Work out the finished part from the listing and answer in its coordinate system (mm). A direction names the side the tool comes from. Round coordinates to 2 decimals unless told otherwise and drop trailing zeros. Order: outer loops, then holes, each group sorted by start corner. A loop starts at its lowest first (then second) coordinate and runs counter-clockwise, first axis right, second up. Notation, with made-up numbers: M 83.5,2.5 L 129.5,2.5 A20 ccw 129.5,30.5 Z; hole C 65,38 d7. An arc over 180 degrees is marked long. Return JSON: item names as keys, results as strings.
from build123d import *

# Parameters (mm, degrees)
SKETCH_3_R          = 1.6
EXTRUDE_2_DEPTH     = 3
SKETCH_4_W          = 58
SKETCH_4_H          = 3
EXTRUDE_3_DEPTH     = 18
SKETCH_5_R          = 1.75
EXTRUDE_4_DEPTH     = 4
SKETCH_7_R          = 8
CUT_EXTRUDE_2_DEPTH = 50


with BuildPart() as part:
    # 草图3 → 凸台-拉伸2 (new body)
    with BuildSketch(Plane.XY):
        with BuildLine():
            Line((-29, 0), (-29, -5))
            Line((-29, -5), (29, -5))
            Line((29, -5), (29, 0))
            ThreePointArc((29, 0), (24, 5), (19, 0))
            Line((19, 0), (-19, 0))
            ThreePointArc((-19, 0), (-24, 5), (-29, 0))
        make_face()
        with Locations((-24, 0)):
            Circle(SKETCH_3_R, mode=Mode.SUBTRACT)
        with Locations((24, 0)):
            Circle(SKETCH_3_R, mode=Mode.SUBTRACT)
    extrude(amount=EXTRUDE_2_DEPTH)

    # 草图4 → 凸台-拉伸3 (add)
    with BuildSketch(Plane.XY.offset(3)):
        with Locations((0, -6.5)):
            Rectangle(SKETCH_4_W, SKETCH_4_H)
    extrude(amount=-EXTRUDE_3_DEPTH)

    # 草图5 → 凸台-拉伸4 (add)
    with BuildSketch(Plane(origin=(29, 0, 0), x_dir=(0, 0, -1), z_dir=(1, 0, 0))):
        with BuildLine():
            Line((-3, -8), (-3, -14))
            ThreePointArc((-3, -14), (6, -23), (15, -14))
            Line((15, -14), (15, -8))
            Line((15, -8), (-3, -8))
        make_face()
        with Locations((6, -14)):
            Circle(SKETCH_5_R, mode=Mode.SUBTRACT)
    extrude_4 = extrude(amount=-EXTRUDE_4_DEPTH)

    # 镜向1: 凸台-拉伸4 across plane
    add(extrude_4.mirror(Plane(origin=(0, 0, 0), x_dir=(0, 0, 1), z_dir=(1, 0, 0))))

    # 草图7 → 切除-拉伸2 (cut)
    with BuildSketch(Plane.ZY.offset(-25)):
        with Locations((-6, -14)):
            Circle(SKETCH_7_R)
    extrude(amount=CUT_EXTRUDE_2_DEPTH, mode=Mode.SUBTRACT)


solid = part.part
Item 1: Find section C-C (y = -18.25). Determine the outline of the cut face in (x, z).
Output:
{"outline": "M -29,-13.93 L -25,-13.93 L -25,1.93 L -29,1.93 Z; M 25,-13.93 L 29,-13.93 L 29,1.93 L 25,1.93 Z"}
Item 2: Consider line 1 along X through (y, z) = (-13.5, -10); line 2 along Y through (x, z) = (-24, 0.65); line 3 along Y through (x, z) = (-26.95, -6). Determine where each line is inside the solid, lowest interval first. Write a range as [from, to].
Output:
{"line 1": "x = [-29, -25], [25, 29]", "line 2": "y = [-8, -1.6], [1.6, 5]", "line 3": "y = [-23, -15.75], [-12.25, -5]"}
Item 3: Find section B-B (x = -24). Determine the outline of the cut face in (y, z).
Output:
{"outline": "M -8,-15 L -5,-15 L -5,0 L -1.6,0 L -1.6,3 L -8,3 L -8,-0.71 A8 cw -8,-11.29 Z; M 1.6,0 L 5,0 L 5,3 L 1.6,3 Z"}
Item 4: Each of these flat-tipped pins is pushed along its axis until it touches: pin 1 (3 mm diameter, centred on x = 5, z = -13, fed in from -Y); pin 2 (1.9 mm diameter, centred on x = 24, y = 0, fed in from +Z); pin 3 (5 mm diameter, centred on x = -11.5, z = -5.5, fed in from +Y); pin 4 (8 mm diameter, centred on x = 8, y = 1, fed in from -Z). Where does it stop, or does it pass through?
Output:
{"pin 1": "stops at y = -8", "pin 2": "passes through", "pin 3": "stops at y = -5", "pin 4": "stops at z = 0"}
Item 5: Which of the six approach directions +Z, -Z, +X, -X, +Y, -Y give full straight-line access (tool end or side, diameter ignored) to faces 1 (the flat face through (29, -11, -6)), 2 (the flat face through (0, -8, -13)), 3 (the flat face through (0, -5, -7)), 4 (the cylindrical face through (-27.028, -12.265, -5.772)), 5 (the flat face through (0, 0, 1))?
Output:
{"face 1": "+Z, -Z, +X, +Y, -Y", "face 2": "+Z, -Z, -Y", "face 3": "-Z, +X, -X, +Y", "face 4": "+X, -X", "face 5": "+Z, -Z, +Y"}
Item 6: The mould has two halves that part along X. Classify faces 6 (the flat face through (0, -8, 1)), 7 (the flat face through (-29, -11, -6)), 8 (the flat face through (0, -4, 3)), 9 (the cylindrical face through (22.82, 1.08, 1.48)): pulls with the +X half, pulls with the -X half, needs draft (parallel to the pull), parting line crosses it, or undercut.
Output:
{"face 6": "undercut", "face 7": "pulls with the -X half", "face 8": "needs draft", "face 9": "undercut"}
Item 7: Find section A-A (z = -6). Determine the outline of the cut face in (x, y).
Output:
{"outline": "M -29,-23 L -25,-23 L -25,-15.75 L -29,-15.75 Z; M -29,-12.25 L -25,-12.25 L -25,-6 L 25,-6 L 25,-12.25 L 29,-12.25 L 29,-5 L -29,-5 Z; M 25,-23 L 29,-23 L 29,-15.75 L 25,-15.75 Z"}
Item 8: Find section D-D (z = 1.25). Determine the outline of the cut face in (x, y), plus the area to 3 significant figures.
Output:
{"outline": "M -29,-19.33 L -25,-19.33 L -25,-8 L 25,-8 L 25,-19.33 L 29,-19.33 L 29,0 A5 ccw 19,0 L -19,0 A5 ccw -29,0 Z; hole C -24,0 d3.2; hole C 24,0 d3.2", "area": "617 mm^2"}
